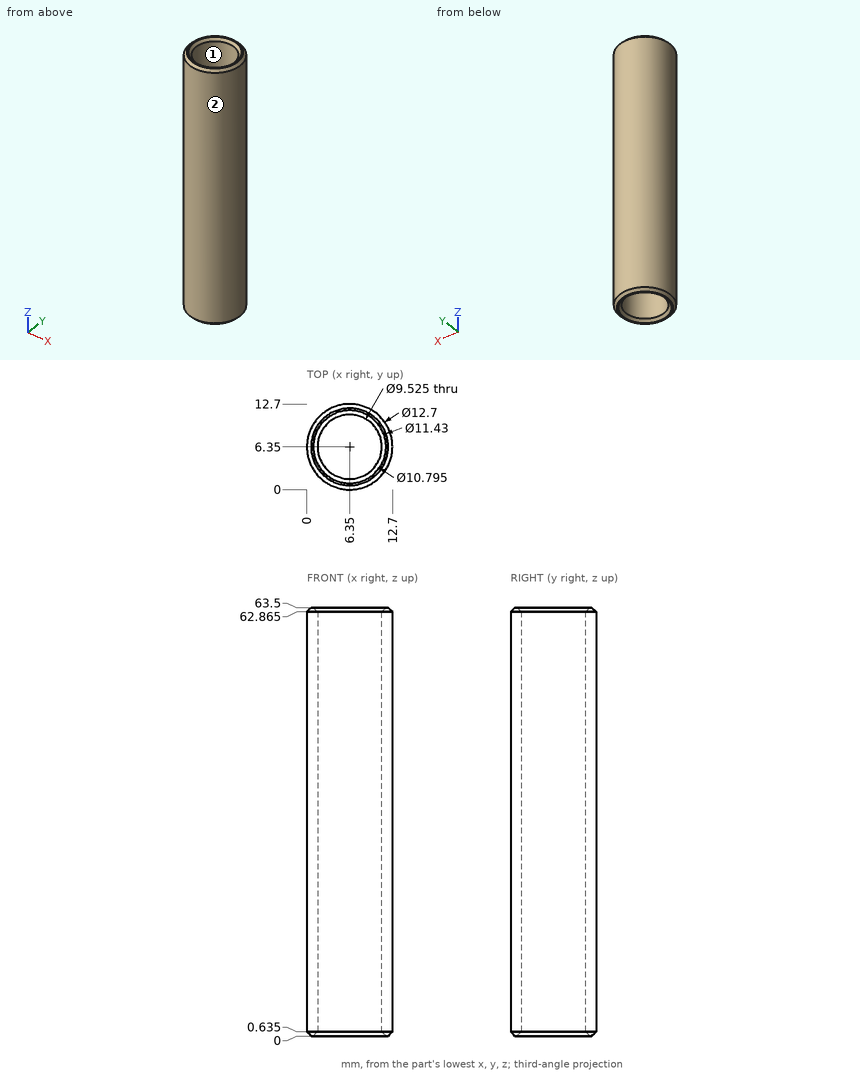
Here's the drawing with two shaded views (mm, measured from the low corner). I have some questions. Give positions to 0.01 mm unless a question says otherwise; leave off trailing zeros. One line per item, written item: value.
Q1. We'd pull the mould along X, two halves only. Please class the marked faces 1 and 2: pulls with the +X half, pulls with the -X half, needs draft (parallel to the pull), parting line crosses it, or undercut.
Answers follow:
face 1: undercut
face 2: parting line crosses it
Q2. If I drill on line 1 along Y through (x, z) = (6.35, 32); line 2 along Y through (x, z) = (5.5, 40), over which ranges is the centre line in solid material (lowest first)?
Answers follow:
line 1: 0 to 1.59, 11.11 to 12.7
line 2: 0.06 to 1.66, 11.04 to 12.64
Q3. I'm going to push flat-ended pins straight in: pin 1 Ø6 at (x, y) = (5.5, 5) entering from +Z; pin 2 Ø3 at (y, z) = (9, 11) entering from -X (3 decimals); pin 3 Ø5 at (x, z) = (1.5, 52) entering from +Y; pin 4 Ø5 at (x, y) = (7, 3) entering from +Z. Where does each tip first touch, or does it pass through?
Answers follow:
pin 1: through
pin 2: x = 0.105
pin 3: y = 12.25
pin 4: z = 63.5
